```python
from build123d import *

# Parameters (mm, degrees)
SKETCH1_W           = 52.8
SKETCH1_H           = 29.8
BOSS_EXTRUDE1_DEPTH = 2
BOSS_EXTRUDE2_DEPTH = 26


with BuildPart() as part:
    # Sketch1 → Boss-Extrude1 (new body)
    with BuildSketch(Plane(origin=(0, 0, 0), x_dir=(1, 0, 0), z_dir=(0, 1, 0))):
        with Locations((26.4, -14.9)):
            Rectangle(SKETCH1_W, SKETCH1_H)
    extrude(amount=BOSS_EXTRUDE1_DEPTH)

    # Sketch2 → Boss-Extrude2 (add)
    with BuildSketch(Plane(origin=(0, 2, 0), x_dir=(1, 0, 0), z_dir=(0, 1, 0))):
        Polygon((0, -27.8), (0, -29.8), (52.8, -29.8), (52.8, 0), (18, 0), (18, -2), (50.8, -2), (50.8, -27.8), align=None)
    extrude(amount=BOSS_EXTRUDE2_DEPTH)


solid = part.part
```
Geometry check sheet. Reference: the model listing, model coordinates, mm. A direction names the side the tool comes from. Give positions to 0.01 mm unless a question says otherwise; leave off trailing zeros. Order: outer loops, then holes, each group sorted by start corner. A loop starts at its lowest first (then second) coordinate and runs counter-clockwise, first axis right, second up. Notation, with made-up numbers: (60, -31.75) - (114, -31.75) arc R12 cw to (114, -13.75) - close; hole circle Ø8 at (8.5, 72.25). An arc over 180 degrees is marked (long way). Write item = value, one per line. Start each with the question number.
1) Section check C-C (z = 20.5). Enter the section's corners in (x, y), then the cut area to 3 significant figures.
2) Gauge pin test, flat ends, axial feed: pin 1 Ø1 at (x, z) = (45.5, 13) entering from -Y; pin 2 Ø13 at (y, z) = (20.5, 19.5) entering from -X; pin 3 Ø2 at (y, z) = (21.5, 1) entering from -X; pin 4 Ø14 at (x, z) = (21, 13.5) entering from +Y. Record the tip position at first contact, or that the pin passes through.
3) Section check D-D (x = 6). Enter the section's corners in (y, z), then the cut area to 3 significant figures.
4) Draft check along Z on faces 4 (the flat face through (26, 14, 29.8)), 5 (the flat face through (25, 2, 14)), 6 (the flat face through (0, 1, 21)). Enter one of: released by +Z, released by -Z, zero draft, split by the parting line, or undercut.
5) Section check A-A (y = 24). Enter the section's corners in (x, z), then the cut area to 3 significant figures.
6) Access from +Z, -Z, +X, -X, +Y, -Y to the whole of each face (thin tool, end or side, straight path). Record for faces 1 (the flat face through (50.8, 15, 15)), 2 (the flat face through (34, 28, 28)), 3 (the flat face through (18, 15, 1)).
7) Section check B-B (x = 20). Enter the section's corners in (y, z), then the cut area to 3 significant figures.
8) Scan lines: L1, parallel to Z at x = 26, y = 20.5; L2, parallel to X at y = 15.25, z = 18.5; L3, parallel to Z at x = 13, y = 16.75. Record each from-to range of solid material in increasing order.
Geometry check:
q1.outline = (0, 0) - (52.8, 0) - (52.8, 28) - (50.8, 28) - (50.8, 2) - (0, 2) - close
q1.area = 158 mm2
q2.pin_1 = 0
q2.pin_2 = 50.8
q2.pin_3 = 18
q2.pin_4 = 2
q3.outline = (0, 0) - (2, 0) - (2, 27.8) - (28, 27.8) - (28, 29.8) - (0, 29.8) - close
q3.area = 112 mm2
q4.face_4 = released by +Z
q4.face_5 = undercut
q4.face_6 = zero draft
q5.outline = (0, 27.8) - (50.8, 27.8) - (50.8, 2) - (18, 2) - (18, 0) - (52.8, 0) - (52.8, 29.8) - (0, 29.8) - close
q5.area = 227 mm2
q6.face_1 = -X, +Y
q6.face_2 = +Z, -Z, +X, -X, +Y
q6.face_3 = -Z, -X, +Y
q7.outline = (0, 0) - (28, 0) - (28, 2) - (2, 2) - (2, 27.8) - (28, 27.8) - (28, 29.8) - (0, 29.8) - close
q7.area = 164 mm2
q8.L1 = 0 to 2, 27.8 to 29.8
q8.L2 = 50.8 to 52.8
q8.L3 = 27.8 to 29.8
